Drawing for the job (mm, zero at the part's lowest x, y, z). Round coordinates to 2 decimals unless told otherwise and drop trailing zeros. Write each loop counter-clockwise with the first axis right and the second up, starting at its lowest first coordinate (ties: lowest second). Pieces come first, ordered by that corner, then holes.
Item 1: Band-saw the part on B-B, the plane x = 24.13. Write the cut outline in (y, z) (1 decimal).
Item 2: Band-saw the part on A-A, the plane z = 12.7. Write the cut outline in (x, y) (1 decimal).
Item 3: Wall check: probe 1 along X at (y, z) = (6.25, 12.7); probe 2 along X at (y, z) = (10.75, 12); probe 3 along Z at (x, y) = (227.33, 10). Give the ranges that are in metal, low to high.
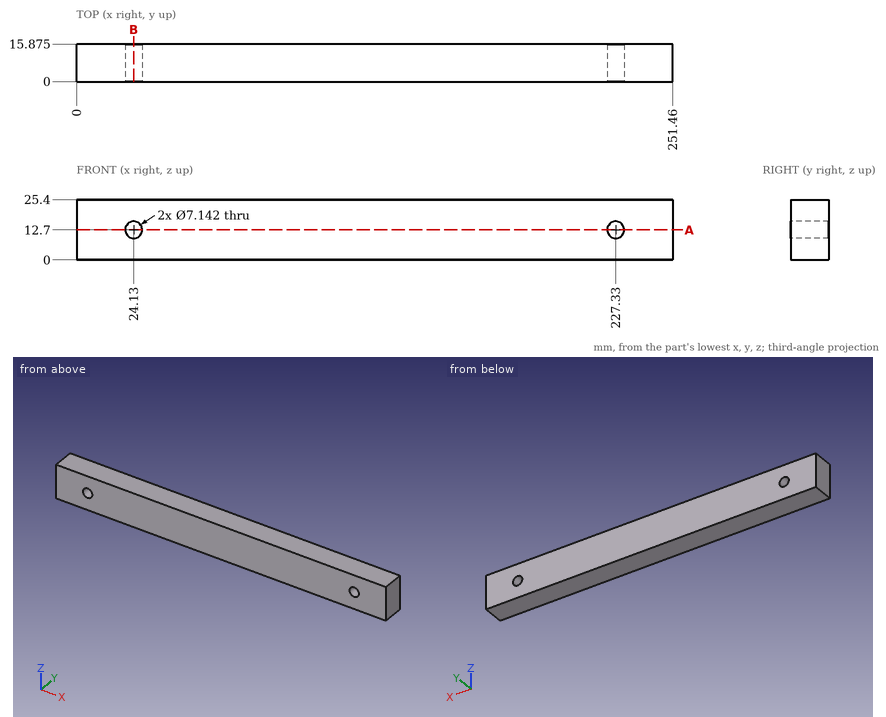
Results:
1. outline: (0, 0) - (15.9, 0) - (15.9, 9.1) - (0, 9.1) - close; (0, 16.3) - (15.9, 16.3) - (15.9, 25.4) - (0, 25.4) - close
2. outline: (0, 0) - (20.6, 0) - (20.6, 15.9) - (0, 15.9) - close; (27.7, 0) - (223.8, 0) - (223.8, 15.9) - (27.7, 15.9) - close; (230.9, 0) - (251.5, 0) - (251.5, 15.9) - (230.9, 15.9) - close
3. probe 1: x = 0 to 20.56, 27.7 to 223.76, 230.9 to 251.46
3. probe 2: x = 0 to 20.63, 27.63 to 223.83, 230.83 to 251.46
3. probe 3: z = 0 to 9.13, 16.27 to 25.4
